from build123d import *

# Parameters (mm, degrees)
SKETCH_1_R               = 39.827146721
SKETCH_1_R_2             = 20.192313572
SKETCH_1_R_3             = 6.968422522
EXTRUDE_1_DEPTH          = 10
EXTRUDE_4_DEPTH          = 25
EXTRUDE_4_DEPTH_BACK     = 10
SKETCH_9_W               = 5.512948522
SKETCH_9_H               = 19.029248926
SKETCH_9_W_2             = 5.494108899
SKETCH_9_H_2             = 10
EXTRUDE_5_DEPTH          = 10
EXTRUDE_5_DEPTH_BACK     = 25
SKETCH_10_W              = 5.512948523
SKETCH_10_H              = 19.029248926
SKETCH_10_W_2            = 5.494108899
SKETCH_10_H_2            = 10
CUT_EXTRUDE_3_DEPTH      = 30
CUT_EXTRUDE_3_DEPTH_BACK = 30
SKETCH_11_R              = 6.215767845
SKETCH_11_W              = 17.292355096
SKETCH_11_H              = 5.512218416


with BuildPart() as part:
    # 草图1 → 凸台-拉伸1 (new body)
    with BuildSketch(Plane.XY):
        Circle(SKETCH_1_R)
        Circle(SKETCH_1_R_2, mode=Mode.SUBTRACT)
        with Locations((0, 30.769644044)):
            Circle(SKETCH_1_R_3, mode=Mode.SUBTRACT)
        with Locations((0, -30.769644044)):
            Circle(SKETCH_1_R_3, mode=Mode.SUBTRACT)
        with Locations((-30.769644044, 0)):
            Circle(SKETCH_1_R_3, mode=Mode.SUBTRACT)
    extrude(amount=EXTRUDE_1_DEPTH)

    # 草图9 → 凸台-拉伸4 (add, two sides: drawn at the far end of the back side and taken through both)
    # profile 1 of 2: a face of its own
    with BuildSketch(Plane(origin=(0, 20, 0), x_dir=(1, 0, 0), z_dir=(0, 1, 0)).offset(-EXTRUDE_4_DEPTH_BACK)):
        with Locations((37.067708268, -4.794824214)):
            Rectangle(SKETCH_9_W, SKETCH_9_H)
        with BuildLine():
            ThreePointArc((35.447720425, -7.685496918), (36.952141211, -9.189917704), (38.456561997, -7.685496918))
            Line((38.456561997, -7.685496918), (38.456561997, -2.475743455))
            ThreePointArc((38.456561997, -2.475743455), (36.952141211, -0.971322669), (35.447720425, -2.475743455))
            Line((35.447720425, -2.475743455), (35.447720425, -7.685496918))
        make_face(mode=Mode.SUBTRACT)
    # profile 2 of 2: a face of its own
    with BuildSketch(Plane(origin=(0, 20, 0), x_dir=(1, 0, 0), z_dir=(0, 1, 0)).offset(-EXTRUDE_4_DEPTH_BACK)):
        with Locations((31.564179558, -4.999991318)):
            Rectangle(SKETCH_9_W_2, SKETCH_9_H_2)
    extrude(amount=EXTRUDE_4_DEPTH + EXTRUDE_4_DEPTH_BACK)

    # 草图10 → 凸台-拉伸5 (add, two sides: drawn at the far end of the back side and taken through both)
    # profile 1 of 2: a face of its own
    with BuildSketch(Plane(origin=(0, -20, 0), x_dir=(1, 0, 0), z_dir=(0, 1, 0)).offset(-EXTRUDE_5_DEPTH_BACK)):
        with Locations((37.067757535, -4.794829971)):
            Rectangle(SKETCH_10_W, SKETCH_10_H)
        with BuildLine():
            ThreePointArc((35.447769691, -7.685502675), (36.952190477, -9.189923461), (38.456611263, -7.685502675))
            Line((38.456611263, -7.685502675), (38.456611263, -2.475749212))
            ThreePointArc((38.456611263, -2.475749212), (36.952190477, -0.971328426), (35.447769691, -2.475749212))
            Line((35.447769691, -2.475749212), (35.447769691, -7.685502675))
        make_face(mode=Mode.SUBTRACT)
    # profile 2 of 2: a face of its own
    with BuildSketch(Plane(origin=(0, -20, 0), x_dir=(1, 0, 0), z_dir=(0, 1, 0)).offset(-EXTRUDE_5_DEPTH_BACK)):
        with Locations((31.564228824, -4.999997076)):
            Rectangle(SKETCH_10_W_2, SKETCH_10_H_2)
    extrude(amount=EXTRUDE_5_DEPTH + EXTRUDE_5_DEPTH_BACK)

    # 草图11 → 切除-拉伸3 (cut, two sides: drawn at the far end of the back side and taken through both)
    with BuildSketch(Plane.XY.offset(-CUT_EXTRUDE_3_DEPTH_BACK)):
        with BuildLine():
            ThreePointArc((39.615066117, 4.486072646), (37.701733016, -0.005715671), (39.62332367, -4.493977606))
            Line((39.62332367, -4.493977606), (43.917498233, -4.493977606))
            Line((43.917498233, -4.493977606), (43.917498233, -6.215767845))
            ThreePointArc((43.917498233, -6.215767845), (48.312709827, -4.395211593), (50.133266078, 0))
            ThreePointArc((50.133266078, 0), (48.429223467, 4.275523982), (44.251416636, 6.206792118))
            Line((44.251416636, 6.206792118), (44.251416636, 4.486072646))
            Line((44.251416636, 4.486072646), (39.615066117, 4.486072646))
        make_face()
        with Locations((43.917498233, 0)):
            Circle(SKETCH_11_R)
        with Locations((35.605239088, 7.242181854)):
            Rectangle(SKETCH_11_W, SKETCH_11_H)
        with Locations((35.271320685, -7.250086814)):
            Rectangle(SKETCH_11_W, SKETCH_11_H)
    extrude(amount=CUT_EXTRUDE_3_DEPTH + CUT_EXTRUDE_3_DEPTH_BACK, mode=Mode.SUBTRACT)


solid = part.part
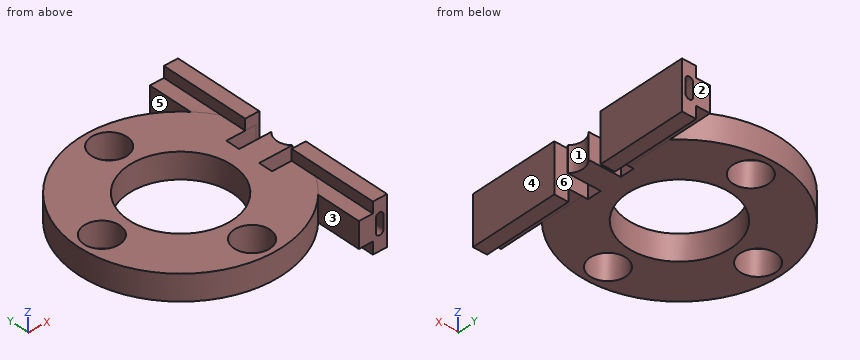
Source: CAD feature listing. Evaluate the final solid. Frame: model axes, mm. Face numbers are marked on the shaded views. A direction names the side the tool comes from. Round coordinates to 2 decimals unless told otherwise and drop trailing zeros. Write each loop counter-clockwise with the first axis right and the second up, starting at its lowest first coordinate (ties: lowest second). Pieces come first, ordered by that corner, then holes. Notation, with made-up numbers: (34.5, 69) - (73.5, 69) arc R17 cw to (73.5, 96) - close; hole circle Ø10 at (57, -29). An arc over 180 degrees is marked (long way). Use CSV: the item, a comma, the result in double quotes. Start each with the question number.
(1) First-contact query: pin 1 Ø11 at (y, z) = (21, 4.5) entering from -X; pin 2 Ø4 at (x, y) = (4.5, -35.5) entering from +Z; pin 3 Ø1.5 at (x, z) = (-29.5, 12) entering from -Y; pin 4 Ø2.5 at (x, y) = (31.5, 22.5) entering from -Z. Flat tips, straight axial feed; report the tip coordinate or a pass-through.
(2) Cut plane A-A, the plane x = 0. Return loops of the section in (y, z).
(3) Material intervals for probe 1 along Y at (x, z) = (0, 6.5); probe 2 along Y at (x, z) = (2.5, 6.75); probe 3 along X at (y, z) = (-3, 1.25), sorted ascending. Write a range as [from, to].
(4) Cut plane B-B, the plane y = 0. Return loops of the section in (x, z).
(5) Cut plane C-C, the plane z = 13.25. Return loops of the section in (x, y).
(6) Set-up query: the marked faces 4, 5 and 6. Return all of +Z, -Z, +X, -X, +Y, -Y with unobstructed straight access to the full face (end or side cutting, diameter ignored); none if empty.
(7) Mould query, pull axis Y, two halves, no side actions, for the marked faces 1, 2 and 3. Classes: pulls with the +Y half, pulls with the -Y half, needs draft (parallel to the pull), parting line crosses it, or undercut.
(8) Cut plane D-D, the plane y = 29.5. Return loops of the section in (x, z), and give its area (3 significant figures).
Geometry says:
1,pin 1,"x = -36.69"
1,pin 2,"z = 10"
1,pin 3,"through"
1,pin 4,"z = 0"
2,outline,"(-39.83, 0) - (-37.74, 0) - (-37.74, 10) - (-39.83, 10) - close; (-23.8, 0) - (-20.19, 0) - (-20.19, 10) - (-23.8, 10) - close; (20.19, 0) - (23.8, 0) - (23.8, 10) - (20.19, 10) - close; (37.74, 0) - (39.83, 0) - (39.83, 10) - (37.74, 10) - close"
3,probe 1,"[-39.83, -37.74], [-23.8, -20.19], [20.19, 23.8], [37.74, 39.83]"
3,probe 2,"[-39.75, -37.27], [-24.27, -20.04], [20.04, 24.27], [37.27, 39.75]"
3,probe 3,"[-39.71, -37.06], [-24.48, -19.97], [19.97, 38.47]"
4,outline,"(-39.83, 0) - (-37.74, 0) - (-37.74, 10) - (-39.83, 10) - close; (-23.8, 0) - (-20.19, 0) - (-20.19, 10) - (-23.8, 10) - close; (20.19, 0) - (37.7, 0) - (37.7, 10) - (20.19, 10) - close"
5,outline,"(34.31, -45) - (39.82, -45) - (39.82, -10.01) - (34.31, -10.01) - close; (34.31, 10) - (39.82, 10) - (39.82, 45) - (34.31, 45) - close"
6,face 4,"+Z, -Z, +X, +Y, -Y"
6,face 5,"+Z, -Z, +Y"
6,face 6,"+Z, -Z, +X"
7,face 1,"undercut"
7,face 2,"pulls with the +Y half"
7,face 3,"needs draft"
8,outline,"(-26.76, 0) - (-6.85, 0) - (-6.85, 10) - (-26.76, 10) - close; (6.85, 0) - (26.76, 0) - (26.76, 10) - (6.85, 10) - close; (28.82, 0) - (34.31, 0) - (34.31, -4.72) - (39.82, -4.72) - (39.82, 14.31) - (34.31, 14.31) - (34.31, 10) - (28.82, 10) - close; hole (35.45, 2.48) arc R1.5 ccw to (38.46, 2.48) - (38.46, 7.69) arc R1.5 ccw to (35.45, 7.69) - close"
8,area,"535 mm²"
